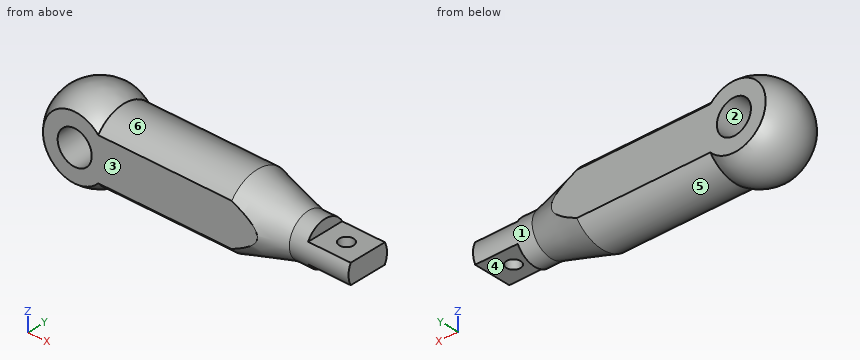
from build123d import *

# Parameters (mm, degrees)
F2_W          = 381
F2_H          = 102.1967058976
F3_DEPTH      = 381.001
F3_DEPTH_BACK = 381.001
F5_DEPTH      = 2771.6493650208
F6_R          = 152.4
F7_DEPTH      = 508.001
F8_R          = 63.5
F9_DEPTH      = 469.901


with BuildPart() as f1:
    # F0 (on Front) → F1 (revolve)
    with BuildSketch(Plane.XZ):
        with BuildLine():
            ThreePointArc((210.6056741876, 317.5), (-180.1669200138, 335.7095186806), (-381, 0))
            Line((-381, 0), (1644.6669101715, 0))
            Line((1644.6669101715, 0), (1709.2056741876, 0))
            Line((1709.2056741876, 0), (2390.6483650208, 0))
            Line((2390.6483650208, 0), (2390.6483650208, 190.5))
            Line((2390.6483650208, 190.5), (1861.6056741876, 190.5))
            Line((1861.6056741876, 190.5), (1404.4056741876, 317.5))
            Line((1404.4056741876, 317.5), (210.6056741876, 317.5))
        make_face()
    revolve(axis=Axis((1529.9751758575, 0, 0), (1, 0, 0)))

    # F2 (on Front) → F3 (cut, two sides)
    with BuildSketch(Plane.XZ) as f3_sk:
        with Locations((2200.1483650208, 139.9983529488)):
            Rectangle(F2_W, F2_H)
        with Locations((2200.1483650208, -139.9983529488)):
            Rectangle(F2_W, F2_H)
    extrude(amount=-F3_DEPTH, mode=Mode.SUBTRACT)
    extrude(f3_sk.sketch, amount=F3_DEPTH_BACK, mode=Mode.SUBTRACT)

    # F4 (on face) → F5 (cut, through all)
    with BuildSketch(Plane.YZ.offset(2390.6483650208)):
        with BuildLine():
            Line((-254, -283.9806331425), (-254, 283.9806331425))
            ThreePointArc((-254, 283.9806331425), (-381, 0), (-254, -283.9806331425))
        make_face()
        with BuildLine():
            ThreePointArc((381, 0), (347.8038240158, 155.5425986667), (254, 283.9806331425))
            Line((254, 283.9806331425), (254, -283.9806331425))
            ThreePointArc((254, -283.9806331425), (347.8038240158, -155.5425986667), (381, 0))
        make_face()
    extrude(amount=-F5_DEPTH, mode=Mode.SUBTRACT)

    # F6 (on face) → F7 (cut, through all)
    with BuildSketch(Plane.XZ.offset(254)):
        Circle(F6_R)
    extrude(amount=-F7_DEPTH, mode=Mode.SUBTRACT)

    # F8 (on face) → F9 (cut, through all)
    with BuildSketch(Plane.XY.offset(88.9)):
        with Locations((2200.1483650208, 0)):
            Circle(F8_R)
    extrude(amount=-F9_DEPTH, mode=Mode.SUBTRACT)


solid = f1.part
For this review, take the finished solid that the model builds, in its own axes (mm). Face numbers are marked on the shaded views. A direction names the side the tool comes from. Give positions to 0.01 mm unless a question says otherwise; leave off trailing zeros. Loops run counter-clockwise (first coordinate to the right, second up) from the corner with the lowest first, then second, coordinate; pieces in that order, holes last. Notation, with made-up numbers: M -4.75,79 L 33.25,79 A37 cw 33.25,115 Z; hole C 83.5,1 d8. An arc over 180 degrees is marked long. Put each result on its own line as item: value. Start each with the question number.
(1) Add section D-D, the plane x = 1373.5. Write out the cut boundary in (y, z), then the cut area to 3 significant figures.
(2) Add section C-C, the plane x = 0. Write out the cut boundary in (y, z), then the cut area to 3 significant figures.
(3) For pin 1 (2 mm diameter, centred on y = -180, z = 274, fed in from -X); pin 2 (3 mm diameter, centred on x = 1938, z = 118.5, fed in from -Y); pin 3 (3 mm diameter, centred on y = -52.5, z = 117.5, fed in from -X), all flat-tipped, find the tip position at first contact; note any pin that passes through.
(4) Machinability: for the marked faces 4, 5 and 6, which of the approach directions +Z, -Z, +X, -X, +Y, -Y give a long, thin tool a straight path to every point of the face, cutting with its end or side? Answer none if there is none.
(5) The part is to be moulded in two halves that separate along Z. For the marked faces 1, 2 and 3, say which applies: +Z half, -Z half, draft (parallel to the pull), parting line (faces both ways), or undercut.
(6) Add section A-A, the plane z = 0. Write out the cut boundary in (x, y), then the cut area to 3 significant figures.
(7) Add section B-B, the plane y = 0. Write out the cut boundary in (x, z).
(8) Wall thickness on L1, parallel to Z at x = 0, y = 11.5; L2, parallel to Z at x = 287.5, y = -5.5; L3, parallel to X at y = -0.5, z = -74.5: over which ranges is each line inside the solid? List them lowest first.
Result:
1. outline: M -254,-190.5 A317.5 ccw 254,-190.5 L 254,190.5 A317.5 ccw -254,190.5 Z
1. area: 284,000 mm^2
2. outline: M -254,-283.98 A381 ccw 254,-283.98 L 254,-152.4 L -254,-152.4 Z; M -254,152.4 L 254,152.4 L 254,283.98 A381 ccw -254,283.98 Z
2. area: 201,000 mm^2
3. pin 1: stops at x = -195.81
3. pin 2: stops at y = -150.34
3. pin 3: stops at x = -359.14
4. face 4: -Z, +X, +Y, -Y
4. face 5: -Z, +X
4. face 6: +Z, +X
5. face 1: parting line
5. face 2: undercut
5. face 3: draft
6. outline: M -283.98,-254 L -152.4,-254 L -152.4,254 L -283.98,254 A381 ccw Z; M 152.4,-254 L 1633.01,-254 L 1861.61,-190.5 L 2390.65,-190.5 L 2390.65,190.5 L 1861.61,190.5 L 1633.01,254 L 152.4,254 Z; hole C 2200.15,0 d127
6. area: 1,140,000 mm^2
7. outline: M 210.61,-317.5 L 1404.41,-317.5 L 1861.61,-190.5 L 2009.65,-190.5 L 2009.65,-88.9 L 2136.65,-88.9 L 2136.65,88.9 L 2009.65,88.9 L 2009.65,190.5 L 1861.61,190.5 L 1404.41,317.5 L 210.61,317.5 A381 ccw long Z; M 2263.65,-88.9 L 2390.65,-88.9 L 2390.65,88.9 L 2263.65,88.9 Z; hole C 0,0 d304.8
8. L1: z = -380.83 to -152.4, 152.4 to 380.83
8. L2: z = -317.45 to 317.45
8. L3: x = -373.64 to -132.95, 132.95 to 2136.65, 2263.65 to 2390.65
